Input: part model. Units: mm. Frame: model coordinates. A direction names the side the tool comes from. Give positions to 0.01 mm unless a question says otherwise; leave off trailing zeros. One line per item, written item: value.
from build123d import *

# Parameters (mm, degrees)
F0_W     = 650
F0_H     = 325
F1_DEPTH = 19
F2_W     = 2
F2_H     = 19
F3_DEPTH = 330
F4_W     = 2
F4_H     = 19
F5_DEPTH = 100


with BuildPart() as f1:
    # F0 (on Top) → F1 (new body)
    with BuildSketch(Plane.XY):
        Rectangle(F0_W, F0_H)
    extrude(amount=F1_DEPTH)

    # F2 (on face) → F3 (cut)
    with BuildSketch(Plane(origin=(-325, 0, 0), x_dir=(0, -1, 0), z_dir=(-1, 0, 0))):
        with Locations((-161.5, 9.5)):
            Rectangle(F2_W, F2_H)
    extrude(amount=-F3_DEPTH, mode=Mode.SUBTRACT)

    # F4 (on face) → F5 (cut)
    with BuildSketch(Plane(origin=(0, 160.5, 0), x_dir=(-1, 0, 0), z_dir=(0, 1, 0))):
        with Locations((0, 9.5)):
            Rectangle(F4_W, F4_H)
    extrude(amount=-F5_DEPTH, mode=Mode.SUBTRACT)


solid = f1.part
Item 1: Access query for faces 1 (the face through (-1, 111, 9)), 2 (the face through (-5, 2, 0)), 3 (the face through (-165, 160.5, 9)). Directions: +Z, -Z, +X, -X, +Y, -Y. A direction counts if a zero-diameter tool reaches every point of the face in a straight line with its end or side. Return the directions, or none.
Verdict:
face 1: +Z, -Z, +Y
face 2: -Z, +X, -X, +Y, -Y
face 3: +Z, -Z, -X, +Y
Item 2: Draft query along X for faces 4 (the face through (-5, 2, 19)), 5 (the face through (1, 111, 9)), 6 (the face through (325, -2, 9)). Return one class per face: pulls with the +X half, pulls with the -X half, needs draft (parallel to the pull), parting line crosses it, or undercut.
Verdict:
face 4: needs draft
face 5: undercut
face 6: pulls with the +X half
Item 3: Pin query (flat end, axial travel): P1, Ø9.5, axis at x = -152.5, z = 11.5, coming from the +Y side; P2, Ø12, axis at x = -47.5, y = -10, coming from the -Z side; P3, Ø0.6, axis at y = 161, z = 6, coming from the -X side. Return the tip coordinate at first contact, or that it passes through.
Verdict:
P1: stops at y = 160.5
P2: stops at z = 0
P3: stops at x = 5
Item 4: Material intervals for L1, parallel to X at y = 146, z = 10.5; L2, parallel to Y at x = -156.5, z = 2, sorted ascending.
Verdict:
L1: x = -325 to -1, 1 to 325
L2: y = -162.5 to 160.5
